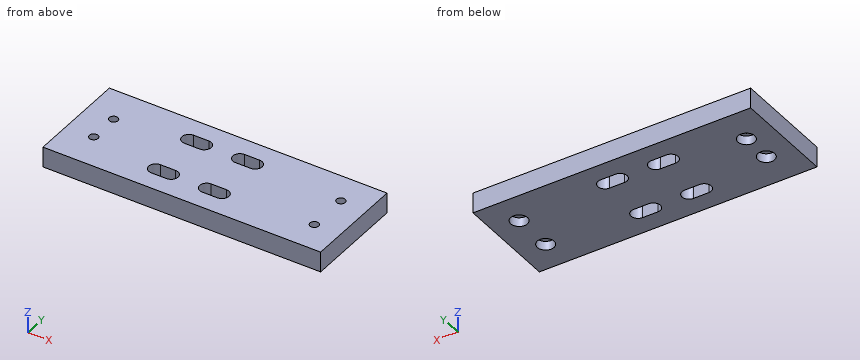
```python
from build123d import *

# Parameters (mm, degrees)
SKETCH1_W           = 109.1
SKETCH1_H           = 40
SKETCH1_R           = 1.7
BOSS_EXTRUDE1_DEPTH = 8
SKETCH2_R           = 3.3
CUT_EXTRUDE1_DEPTH  = 3.5


with BuildPart() as part:
    # Sketch1 → Boss-Extrude1 (new body)
    with BuildSketch(Plane.XY.offset(238)):
        with Locations((281.75, 300)):
            Rectangle(SKETCH1_W, SKETCH1_H)
        with Locations((238, 294)):
            Circle(SKETCH1_R, mode=Mode.SUBTRACT)
        with Locations((238, 306)):
            Circle(SKETCH1_R, mode=Mode.SUBTRACT)
        with Locations((326, 292)):
            Circle(SKETCH1_R, mode=Mode.SUBTRACT)
        with Locations((326, 308)):
            Circle(SKETCH1_R, mode=Mode.SUBTRACT)
        with BuildLine():
            Line((265, 287.25), (271, 287.25))
            ThreePointArc((271, 287.25), (273.75, 290), (271, 292.75))
            Line((271, 292.75), (265, 292.75))
            ThreePointArc((265, 292.75), (262.25, 290), (265, 287.25))
        make_face(mode=Mode.SUBTRACT)
        with BuildLine():
            Line((265, 307.25), (271, 307.25))
            ThreePointArc((271, 307.25), (273.75, 310), (271, 312.75))
            Line((271, 312.75), (265, 312.75))
            ThreePointArc((265, 312.75), (262.25, 310), (265, 307.25))
        make_face(mode=Mode.SUBTRACT)
        with BuildLine():
            Line((285, 287.25), (291, 287.25))
            ThreePointArc((291, 287.25), (293.75, 290), (291, 292.75))
            Line((291, 292.75), (285, 292.75))
            ThreePointArc((285, 292.75), (282.25, 290), (285, 287.25))
        make_face(mode=Mode.SUBTRACT)
        with BuildLine():
            Line((285, 307.25), (291, 307.25))
            ThreePointArc((291, 307.25), (293.75, 310), (291, 312.75))
            Line((291, 312.75), (285, 312.75))
            ThreePointArc((285, 312.75), (282.25, 310), (285, 307.25))
        make_face(mode=Mode.SUBTRACT)
    extrude(amount=BOSS_EXTRUDE1_DEPTH)

    # Sketch2 → Cut-Extrude1 (cut)
    with BuildSketch(Plane.XY.offset(238)):
        with Locations((238, 294)):
            Circle(SKETCH2_R)
        with Locations((238, 306)):
            Circle(SKETCH2_R)
        with Locations((326, 292)):
            Circle(SKETCH2_R)
        with Locations((326, 308)):
            Circle(SKETCH2_R)
    extrude(amount=CUT_EXTRUDE1_DEPTH, mode=Mode.SUBTRACT)


solid = part.part
```
Geometry check sheet. Reference: the model listing, model coordinates, mm. Coordinates: 2 decimals unless noted, no trailing zeros. Loops run counter-clockwise (first coordinate to the right, second up) from the corner with the lowest first, then second, coordinate; pieces in that order, holes last.
Item 1: Sectioned sample at A-A, the plane x = 326. Record the boundary of the cut face in (y, z), then the cut area to 3 significant figures.
Item 2: Thickness scan on line 1 (Y direction, x = 326, z = 243.9); line 2 (Y direction, x = 238, z = 240.45); line 3 (X direction, y = 306, z = 239.8). Record the ranges inside material, lowest first.
Item 3: Sectioned sample at B-B, the plane z = 244.75. Count the separate pieces of the cut face and the enclosed holes in it, then the cut area to 3 significant figures.
Item 4: Go/stop test with flat-tipped pins: pin 1 Ø8.5 at (x, y) = (238, 294) entering from +Z; pin 2 Ø3.5 at (x, y) = (326.5, 291) entering from -Z; pin 3 Ø2 at (x, y) = (326, 292) entering from -Z. Record where each tip stops, or that it passes through.
Check result:
1. outline: (280, 238) - (288.7, 238) - (288.7, 241.5) - (290.3, 241.5) - (290.3, 246) - (280, 246) - close; (293.7, 241.5) - (295.3, 241.5) - (295.3, 238) - (304.7, 238) - (304.7, 241.5) - (306.3, 241.5) - (306.3, 246) - (293.7, 246) - close; (309.7, 241.5) - (311.3, 241.5) - (311.3, 238) - (320, 238) - (320, 246) - (309.7, 246) - close
1. area: 243 mm2
2. line 1: y = 280 to 290.3, 293.7 to 306.3, 309.7 to 320
2. line 2: y = 280 to 290.7, 297.3 to 302.7, 309.3 to 320
2. line 3: x = 227.2 to 234.7, 241.3 to 323.38, 328.62 to 336.3
3. separate pieces: 1
3. enclosed holes: 8
3. area: 4,100 mm2
4. pin 1: stops at z = 246
4. pin 2: stops at z = 241.5
4. pin 3: passes through
